Geometry: final body of the model. Coordinates: model frame, mm. A direction names the side the tool comes from. Round coordinates to 2 decimals unless told otherwise and drop trailing zeros. Order: outer loops, then holes, each group sorted by start corner. A loop starts at its lowest first (then second) coordinate and runs counter-clockwise, first axis right, second up. Notation, with made-up numbers: M 34.25,63 L 47.25,63 A16 cw 47.25,72 Z; hole C 65,-30.75 d8. An arc over 180 degrees is marked long. Put each result on its own line as item: value. Start each with the question number.
1) Section D-D, the plane z = 26. Return loops of the section in (x, y).
2) First-contact query: P1, Ø10, axis at x = 14, y = -50, coming from the -Z side; P2, Ø10, axis at x = -12.5, y = -34, coming from the -Z side; P3, Ø2, axis at x = -11, z = 13.5, coming from the +Y side. Flat tips, straight axial feed; report the tip coordinate or a pass-through.
3) Section A-A, the plane y = -50. Return loops of the section in (x, z).
4) Material intervals for probe 1 along Y at (x, z) = (15, 26.3); probe 2 along Y at (x, z) = (-7, 19.75); probe 3 along X at (y, z) = (-10, 28.6), sorted ascending. Write a range as [from, to].
5) Section C-C, the plane z = 15. Return loops of the section in (x, y), then the cut area to 3 significant figures.
6) Draft query along Z for faces 6 (the cylindrical face through (-10.55, -22.46, 9.01)), 7 (the flat face through (2, -30, 0)), 8 (the flat face through (0, -12, 15)). Return one class per face: pulls with the +Z half, pulls with the -Z half, needs draft (parallel to the pull), parting line crosses it, or undercut.
7) Section B-B, the plane x = 11.5. Return loops of the section in (y, z).
8) Access query for faces 1 (the flat face through (0, -52, 15)), 2 (the flat face through (25, -10, 27)), 3 (the flat face through (15, -52, 25)), 4 (the flat face through (15, -40, 28)), 5 (the flat face through (0, -30, 15)). Directions: +Z, -Z, +X, -X, +Y, -Y. A direction counts if a zero-diameter tool reaches every point of the face in a straight line with its end or side. Return the directions, or none.
from build123d import *

# Parameters (mm, degrees)
F1_DEPTH  = 20
F4_D      = 3.2
F5_R      = 2.55
F6_DEPTH  = 5
F7_W      = 5
F7_H      = 30
F8_DEPTH  = 5
F10_W     = 20
F10_H     = 20
F10_H_2   = 40
F11_DEPTH = 5
F13_D     = 3.5
F13_DEPTH = 10


with BuildPart() as f1:
    # F0 (on Front) → F1 (new body)
    with BuildSketch(Plane.XZ):
        Polygon((0, 0), (25, 0), (25, 5), (5, 5), (5, 25), (25, 25), (25, 30), (0, 30), align=None)
    extrude(amount=F1_DEPTH)

    # F4 (through all)
    with Locations(Plane(origin=(0, 0, 25), x_dir=(1, 0, 0), z_dir=(0, 0, -1))):
        with Locations((15, 10), (15, -10)):
            Hole(F4_D / 2)

    # F5 (on face) → F6 (join)
    with BuildSketch(Plane.XZ.offset(20)):
        Polygon((5, 30), (0, 30), (0, 0), (5, 0), (5, 5), (5, 25), align=None)
        with BuildLine():
            Line((0, 0), (0, 30))
            Line((0, 30), (-14.910067, 17.235307))
            ThreePointArc((-14.910067, 17.235307), (-17.42027, 10.106411), (-12.494612, 4.374033))
            Line((-12.494612, 4.374033), (0, 0))
        make_face()
        with Locations((-10, 11.5)):
            Circle(F5_R, mode=Mode.SUBTRACT)
    extrude(amount=F6_DEPTH)

    # F7 (on face) → F8 (join)
    with BuildSketch(Plane.XZ.offset(25)):
        with Locations((2.5, 15)):
            Rectangle(F7_W, F7_H)
    extrude(amount=F8_DEPTH)

    # F9: F1 across face


with BuildPart() as f1_1:
    add(f1.part)
    add(f1.part.mirror(Plane(origin=(2.5, -30, 15), x_dir=(1, 0, 0), z_dir=(0, -1, 0))))

    # F10 (on face) → F11 (cut, through all)
    with BuildSketch(Plane.XY.offset(5)):
        with Locations((15, -10)):
            Rectangle(F10_W, F10_H)
        with Locations((15, -40)):
            Rectangle(F10_W, F10_H_2)
    extrude(amount=-F11_DEPTH, mode=Mode.SUBTRACT)

    # F13
    with Locations(Plane(origin=(0, 0, 0), x_dir=(0, -1, 0), z_dir=(-1, 0, 0))):
        with Locations((10, 15), (50, 15)):
            Hole(F13_D / 2, depth=F13_DEPTH)


solid = f1_1.part
Result sheet:
1. outline: M -4.67,-40 L 0,-40 L 0,-60 L 25,-60 L 25,-40 L 5,-40 L 5,-20 L 25,-20 L 25,0 L 0,0 L 0,-20 L -4.67,-20 L -4.67,-25 L 0,-25 L 0,-35 L -4.67,-35 Z; hole C 15,-50 d3.2; hole C 15,-10 d3.2
2. P1: stops at z = 25
2. P2: stops at z = 2.66
2. P3: stops at y = -20
3. outline: M 0,0 L 5,0 L 5,13.25 L 0,13.25 Z; M 0,16.75 L 5,16.75 L 5,25 L 13.4,25 L 13.4,30 L 0,30 Z; M 16.6,25 L 25,25 L 25,30 L 16.6,30 Z
4. probe 1: y = [-60, -51.6], [-48.4, -40], [-20, -11.6], [-8.4, 0]
4. probe 2: y = [-40, -35], [-25, -20]
4. probe 3: x = [0, 13.4], [16.6, 25]
5. outline: M -16.69,-40 L 0,-40 L 0,-48.25 L 5,-48.25 L 5,-11.75 L 0,-11.75 L 0,-20 L -16.69,-20 L -16.69,-25 L 0,-25 L 0,-35 L -16.69,-35 Z; M 0,-60 L 5,-60 L 5,-51.75 L 0,-51.75 Z; M 0,-8.25 L 5,-8.25 L 5,0 L 0,0 Z
5. area: 432 mm2
6. face 6: undercut
6. face 7: pulls with the -Z half
6. face 8: needs draft
7. outline: M -60,25 L -40,25 L -40,30 L -60,30 Z; M -20,25 L 0,25 L 0,30 L -20,30 Z
8. face 1: +Z, -Z, -X, -Y
8. face 2: +Z, -Z, +X, +Y, -Y
8. face 3: -Z, +X, +Y, -Y
8. face 4: +Z, -Z, +X
8. face 5: +Z, -Z, -X
